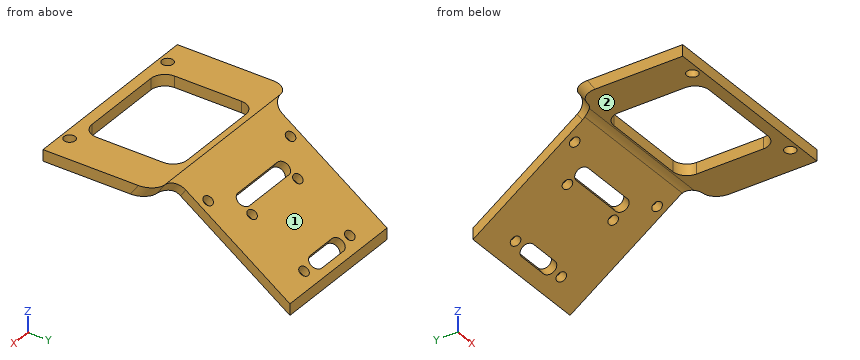
Autodesk Inventor part; units mm, degrees
ref_plane "YZ Plane" through (0, 0, 0) normal (1, 0, 0) x (0, 1, 0)
ref_plane "XZ Plane" through (0, 0, 0) normal (0, 1, 0) x (-1, 0, 0)
ref_plane "XY Plane" through (0, 0, 0) normal (0, 0, 1) x (1, 0, 0)
sketch "Sketch1" plane through (0, 0, 0) normal (0, 0, 1) x (1, 0, 0)
  circle A0 centre (42.125, -15.4) radius 2 construction
  circle A1 centre (-7.875, -15.4) radius 2 construction
  line L0 (-4.825, -12.4) -> (-2.825, -14.4) construction
  line L1 (-9.825, -12.4) -> (-4.825, -12.4) construction
  arc A2 (-14.825, -7.4) -> (-9.825, -12.4) centre (-9.825, -7.4) ccw construction
  line L2 (-14.825, -7.4) -> (-14.825, 13.6) construction
  line L3 (-14.825, 13.6) -> (-15.625, 13.6) construction
  line L4 (-15.625, 13.6) -> (-15.625, 14.6) construction
  line L5 (-14.825, 15.4) -> (-15.625, 14.6) construction
  line L6 (-14.825, 15.4) -> (-14.825, 18.4) construction
  line L7 (-14.825, 18.4) -> (-17.125, 18.4) construction
  line L8 (-17.125, 18.4) -> (-17.125, -18.4) construction
  line L9 (-17.125, -18.4) -> (51.375, -18.4) construction
  line L10 (51.375, 18.4) -> (51.375, -18.4) construction
  line L11 (49.075, 18.4) -> (51.375, 18.4) construction
  line L12 (49.075, 15.4) -> (49.075, 18.4) construction
  line L13 (49.875, 14.6) -> (49.075, 15.4) construction
  line L14 (49.875, 13.6) -> (49.875, 14.6) construction
  line L15 (49.075, 13.6) -> (49.875, 13.6) construction
  line L16 (49.075, -7.4) -> (49.075, 13.6) construction
  arc A3 (44.075, -12.4) -> (49.075, -7.4) centre (44.075, -7.4) ccw construction
  line L17 (39.075, -12.4) -> (44.075, -12.4) construction
  line L18 (37.075, -14.4) -> (39.075, -12.4) construction
  line L19 (37.075, -14.4) -> (-2.825, -14.4) construction
  line L20 (-17.125, -18.4) -> (51.375, -18.4)
  line L21 (51.375, -18.4) -> (51.375, 21.449)
  line L22 (51.375, 21.449) -> (-17.125, 21.449)
  line L23 (-17.125, 21.449) -> (-17.125, -18.4)
  point P0 (0, 0)
extrude "Extrusion1" add sketch "Sketch1" along normal blind 4
sketch "Sketch2" plane through (51.375, -18.4, 0) normal (1, 0, 0) x (0, 0, -1)
  line L0 (0, 0) -> (0, 39.849) construction
  line L1 (0, 39.849) -> (-4, 39.849) construction
  line L2 (-4, 0) -> (-4, 39.849) construction
  line L3 (0, 0) -> (-4, 0) construction
  line L4 (-4, 39.849) -> (24.6788, 80.8066)
  line L5 (24.6788, 80.8066) -> (28.6788, 80.8066)
  line L6 (28.6788, 80.8066) -> (0, 39.849)
  line L7 (-4, 39.849) -> (0, 39.849)
  point P0 (0, 18.4)
  dimension "d2" = 55
  dimension "d5" = 50
extrude "Extrusion2" add sketch "Sketch2" against normal up to surface (68.5 mm away)
sketch "Sketch4" plane through (-17.125, 21.449, 4) normal (0, 0.5735764, 0.819152) x (1, 0, 0)
  line L0 (22.585, 45) -> (45.915, 45) construction
  line L1 (45.915, 45) -> (45.915, 22.57) construction
  line L2 (45.915, 22.57) -> (22.585, 22.57) construction
  line L3 (22.585, 22.57) -> (22.585, 45) construction
  line L4 (68.5, 50) -> (0, 50) construction
  point P0 (17.125, -15.2757)
  point P1 (34.25, 45)
  point P2 (34.25, 50)
  dimension "d11" = 23.33
  dimension "d12" = 22.43
  dimension "d13" = 5
hole "Hole1" at (5.46, 58.3109, -21.8109) at (28.79, 58.3109, -21.8109) at (28.79, 39.9373, -8.9456) at (5.46, 39.9373, -8.9456) direction (0, -0.5735764, -0.819152) diameter 3.5 end through all
sketch "Sketch5" plane through (-17.125, 21.449, 4) normal (0, 0.5735764, 0.819152) x (1, 0, 0)
  circle A0 centre (45.915, 22.57) radius 1.75
  circle A1 centre (22.585, 45) radius 1.75
  circle A2 centre (45.915, 45) radius 1.75
  circle A3 centre (22.585, 22.57) radius 1.75
  line L0 (0, 50) -> (0, 0)
  line L1 (68.5, 0) -> (0, 0)
  line L2 (68.5, 50) -> (68.5, 0)
  line L3 (68.5, 50) -> (0, 50)
  line L4 (28.75, 45) -> (39.75, 45) construction
  line L5 (28.75, 47.5) -> (39.75, 47.5)
  line L6 (39.75, 42.5) -> (28.75, 42.5)
  arc A4 (28.75, 47.5) -> (28.75, 42.5) centre (28.75, 45) ccw
  arc A5 (39.75, 42.5) -> (39.75, 47.5) centre (39.75, 45) ccw
  point P0 (17.125, -15.2757)
  point P1 (34.25, 45)
  dimension "d25" = 23.33
  dimension "d26" = 5
  dimension "d27" = 11
  dimension "d28" = 11.665
extrude "Extrusion3" cut sketch "Sketch5" against normal through all contours L5 A5 L6 A4
sketch "Sketch6" plane through (-17.125, 21.449, 4) normal (0, 0.5735764, 0.819152) x (1, 0, 0)
  line L0 (24.25, 17.57) -> (44.25, 17.57) construction
  line L1 (24.25, 15.07) -> (44.25, 15.07)
  line L2 (44.25, 20.07) -> (24.25, 20.07)
  arc A0 (24.25, 20.07) -> (24.25, 15.07) centre (24.25, 17.57) ccw
  arc A1 (44.25, 15.07) -> (44.25, 20.07) centre (44.25, 17.57) ccw
  line L3 (68.5, 0) -> (0, 0)
  circle A2 centre (22.585, 22.57) radius 1.75
  point P0 (17.125, -15.2757)
  point P1 (34.25, 17.57)
  point P2 (34.25, 0)
  dimension "d31" = 5
  dimension "d32" = 20
  dimension "d33" = 5
extrude "Extrusion4" cut sketch "Sketch6" against normal through all contours A0 L2 A1 L1
sketch "Sketch7" plane through (-17.125, 21.449, 4) normal (0, 0.5735764, 0.819152) x (1, 0, 0)
  line L0 (24.25, 20.07) -> (44.25, 20.07)
  line L1 (68.5, 0) -> (0, 0)
  point P0 (17.125, -15.2757)
  point P1 (13.25, 11.5)
  point P2 (55.25, 11.5)
  point P3 (34.25, 20.07)
  dimension "d36" = 42
  dimension "d37" = 21
  dimension "d45" = 11.5
hole "Hole2" at (-3.875, 30.8693, -2.5961) at (38.125, 30.8693, -2.5961) direction (0, -0.5735764, -0.819152) diameter 3.5 end through all
sketch "Sketch8" plane through (-17.125, 21.449, 4) normal (0, 0.5735764, 0.819152) x (1, 0, 0)
  line L0 (0, 25.2888) -> (68.5, 25.2888) construction
  circle A0 centre (13.25, 11.5) radius 1.75 construction
  circle A1 centre (55.25, 11.5) radius 1.75 construction
  line L1 (24.25, 20.07) -> (44.25, 20.07) construction
  arc A2 (44.25, 15.07) -> (44.25, 20.07) centre (44.25, 17.57) ccw construction
  line L2 (44.25, 15.07) -> (24.25, 15.07) construction
  arc A3 (24.25, 20.07) -> (24.25, 15.07) centre (24.25, 17.57) ccw construction
  arc A4 (28.75, 47.5) -> (28.75, 42.5) centre (28.75, 45) ccw construction
  line L3 (28.75, 47.5) -> (39.75, 47.5) construction
  arc A5 (39.75, 42.5) -> (39.75, 47.5) centre (39.75, 45) ccw construction
  line L4 (39.75, 42.5) -> (28.75, 42.5) construction
  circle A6 centre (45.915, 22.57) radius 1.75 construction
  circle A7 centre (22.585, 45) radius 1.75 construction
  circle A8 centre (45.915, 45) radius 1.75 construction
  circle A9 centre (22.585, 22.57) radius 1.75 construction
  line L5 (0, 50) -> (0, 0) construction
  line L6 (68.5, 0) -> (0, 0) construction
  line L7 (68.5, 50) -> (68.5, 0) construction
  line L8 (68.5, 50) -> (0, 50) construction
  line L9 (0, 0) -> (9.5, 0)
  line L10 (9.5, 0) -> (9.5, 54)
  line L11 (9.5, 54) -> (0, 54)
  line L12 (0, 54) -> (0, 0)
  line L13 (68.5, 0) -> (59, 0)
  line L14 (59, 0) -> (59, 54)
  line L15 (59, 54) -> (68.5, 54)
  line L16 (68.5, 54) -> (68.5, 0)
  point P0 (17.125, -15.2757)
  dimension "d50" = 9.5
  dimension "d51" = 9.5
  dimension "d52" = 4
extrude "Extrusion5" cut sketch "Sketch8" against normal through all
fillet "Fillet1" radius 5 2 edges at (41.875, 20.0486, 2) (-7.625, 20.0486, 2)
sketch "Sketch9" plane through (0, 0, 4) normal (0, 0, 1) x (1, 0, 0)
  line L0 (-15.875, 15.26) -> (50.125, 15.26) construction
  line L1 (50.125, 15.26) -> (50.125, 13.6) construction
  line L2 (-15.875, 13.6) -> (50.125, 13.6) construction
  line L3 (-15.875, 15.26) -> (-15.875, 13.6) construction
  line L4 (-2.825, -14.4) -> (37.075, -14.4) construction
  line L5 (37.075, -14.4) -> (-2.825, -14.4)
  line L6 (-2.825, -14.4) -> (-2.825, 19.26)
  line L7 (-2.825, 19.26) -> (37.075, 19.26)
  line L8 (37.075, 19.26) -> (37.075, -14.4)
  point P0 (0, 0)
  dimension "d54" = 4
extrude "Extrusion6" cut sketch "Sketch9" against normal through all
fillet "Fillet2" radius 5 6 edges at (-2.825, 19.26, 2) (37.075, 19.26, 2) (37.075, -14.4, 2) (-2.825, -14.4, 2) (51.375, 20.0486, 2) (-17.125, 20.0486, 2)
sketch "Sketch10" plane through (0, 0, 4) normal (0, 0, 1) x (1, 0, 0)
  circle A0 centre (-7.875, -15.4) radius 2 construction
  circle A1 centre (42.125, -15.4) radius 2 construction
  point P0 (0, 0)
hole "Hole3" at (-7.875, -15.4, 4) at (42.125, -15.4, 4) direction (0, 0, -1) diameter 4 end through all
fillet "Fillet3" radius 5 1 edges at (17.125, 21.449, 0)
equation "\"d51\" = d50"
properties part number "UserInterface mount"
Geometry check sheet. Reference: the model listing, model coordinates, mm. Face numbers are marked on the shaded views. A direction names the side the tool comes from. Round coordinates to 2 decimals unless told otherwise and drop trailing zeros. Loops run counter-clockwise (first coordinate to the right, second up) from the corner with the lowest first, then second, coordinate; pieces in that order, holes last. Notation, with made-up numbers: M 53,-39 L 73,-39 A19 ccw 73,-5 Z; hole C 58,-17 d11. An arc over 180 degrees is marked long. Return JSON: item names as keys, results as strings. Group by question number.
(1) Section check A-A, the plane y = -15.4. Enter the section's corners in (x, z) (3 decimals).
(2) Section check D-D, the plane x = 21. Enter the section's corners in (y, z), and give its area (3 significant figures).
(3) Go/stop test with flat-tipped pins: pin 1 (8 mm diameter, centred on x = -7.5, y = 26.5, fed in from -Z); pin 2 (8 mm diameter, centred on y = 46.5, z = -9, fed in from +X) (3 decimals); pin 3 (12 mm diameter, centred on x = 10, y = 52.5, fed in from +Z). Record where each tip stops, or that it passes through.
(4) Section check B-B, the plane y = 0.5. Enter the section's corners in (x, z) (3 decimals), and give its area (3 significant figures).
(5) Scan lines: line 1 along X through (y, z) = (-15.4, 1.85) (3 decimals); line 2 along X through (y, z) = (-15, 1) (3 decimals); line 3 along Z through (x, y) = (47, 15.5). Record each from-to range of solid material in increasing order. Write a range as [from, to].
(6) Set-up check for the marked faces 1 and 2: record each of +Z, -Z, +X, -X, +Y, -Y from which the full face is reachable in a straight line by a thin tool's end or side.
(7) Section check C-C, the plane x = -1. Enter the section's corners in (y, z).
Data:
{
 "1": {"outline": "M -17.125,0 L -9.875,0 L -9.875,4 L -17.125,4 Z; M -5.875,0 L 40.125,0 L 40.125,4 L -5.875,4 Z; M 44.125,0 L 51.375,0 L 51.375,4 L 44.125,4 Z"},
 "2": {"outline": "M -18.4,0 L -14.4,0 L -14.4,4 L -18.4,4 Z; M 19.26,0 L 19.87,0 A5 cw 22.74,-0.9 L 31.91,-7.33 L 33.79,-4.64 L 21.45,4 L 19.26,4 Z; M 36.01,-10.2 L 54.38,-23.06 L 56.26,-20.38 L 37.89,-7.51 Z; M 58.48,-25.93 L 62.41,-28.68 L 62.41,-24.68 L 60.36,-23.24 Z", "area": "156 mm²"},
 "3": {"pin 1": "z = -6.34", "pin 2": "x = 41.875", "pin 3": "z = -13.54"},
 "4": {"outline": "M -17.125,0 L -2.825,0 L -2.825,4 L -17.125,4 Z; M 37.075,0 L 51.375,0 L 51.375,4 L 37.075,4 Z", "area": "114 mm²"},
 "5": {"line 1": "[-17.125, -9.875], [-5.875, 40.125], [44.125, 51.375]", "line 2": "[-17.125, -9.835], [-5.915, 40.165], [44.085, 51.375]", "line 3": "[0, 4]"},
 "6": {"face 1": "+Z, +X, -X, +Y", "face 2": "-Z, +X, -X, -Y"},
 "7": {"outline": "M -18.4,0 L -13.26,0 L -13.26,4 L -18.4,4 Z; M 18.12,0 L 19.87,0 A5 cw 22.74,-0.9 L 62.41,-28.68 L 62.41,-24.68 L 21.45,4 L 18.12,4 Z"}
}
